Check sheet for the modelled part. Datum: model origin and axes. Units: mm. Round coordinates to 2 decimals unless told otherwise and drop trailing zeros. Order: outer loops, then holes, each group sorted by start corner. A loop starts at its lowest first (then second) coordinate and runs counter-clockwise, first axis right, second up.
Q1. Cross-section at B-B on x = -35. Record the cut outline in (y, z) (3 decimals), then the cut area to 3 significant figures.
Q2. Depth check by flat-ended pin: P1, Ø18.5, axis at x = 26.5, y = 14, coming from the +Z side. Enter the tip coordinate at first touch or a pass-through.
Q3. Scan lines: probe 1 along X at (y, z) = (-34.5, 3.75); probe 2 along X at (y, z) = (-36, 4.25); probe 3 along Y at (x, z) = (33, 4.75). Record each from-to range of solid material in increasing order.
Q4. Cross-section at A-A on y = 32.5. Record the cut outline in (x, z) (3 decimals).
Q5. Cross-section at C-C on z = 4.5. Give the number of separate pieces and of enclosed holes in the cut face, then the cut area to 3 significant figures.
from build123d import *

# Parameters (mm, degrees)
F1_DEPTH = 6.35
F3_DEPTH = 3.175


with BuildPart() as f1:
    # F0 (on Top) → F1 (new body)
    with BuildSketch(Plane.XY):
        with BuildLine():
            Line((44.45, 50.8), (-44.45, 50.8))
            ThreePointArc((-44.45, 50.8), (-48.940128, 48.940128), (-50.8, 44.45))
            Line((-50.8, 44.45), (-50.8, -44.45))
            ThreePointArc((-50.8, -44.45), (-48.940128, -48.940128), (-44.45, -50.8))
            Line((-44.45, -50.8), (44.45, -50.8))
            ThreePointArc((44.45, -50.8), (48.940128, -48.940128), (50.8, -44.45))
            Line((50.8, -44.45), (50.8, 44.45))
            ThreePointArc((50.8, 44.45), (48.940128, 48.940128), (44.45, 50.8))
        make_face()
    extrude(amount=F1_DEPTH)

    # F2 (on face) → F3 (cut)
    with BuildSketch(Plane.XY.offset(6.35)):
        with BuildLine():
            ThreePointArc((-24.847122, 30.86718), (-8.580237, 34.973614), (7.661782, 30.769903))
            ThreePointArc((7.661782, 30.769903), (-13.391629, 38.003846), (-33.371605, 28.186688))
            ThreePointArc((-33.371605, 28.186688), (-37.418416, 12.612971), (-27.426904, 0))
            ThreePointArc((-27.426904, 0), (-9.473393, 1.300027), (-4.446225, 18.584304))
            ThreePointArc((-4.446225, 18.584304), (-9.355194, 26.176966), (-18.170381, 28.186688))
            ThreePointArc((-18.170381, 28.186688), (-27.074817, 20.28871), (-24.843689, 8.597298))
            ThreePointArc((-24.843689, 8.597298), (-18.2062, 6.472593), (-12.664793, 10.699108))
            ThreePointArc((-12.664793, 10.699108), (-12.67809, 13.468506), (-14.519384, 15.537172))
            ThreePointArc((-14.519384, 15.537172), (-17.08667, 15.877181), (-18.994594, 14.12607))
            ThreePointArc((-18.994594, 14.12607), (-16.63705, 14.888107), (-14.519384, 13.601947))
            ThreePointArc((-14.519384, 13.601947), (-14.784471, 10.552305), (-17.140003, 8.597298))
            ThreePointArc((-17.140003, 8.597298), (-20.512291, 8.645462), (-23.187581, 10.699108))
            ThreePointArc((-23.187581, 10.699108), (-24.847122, 16.641338), (-22.353067, 22.284373))
            ThreePointArc((-22.353067, 22.284373), (-16.15161, 24.669828), (-10.003858, 22.149192))
            ThreePointArc((-10.003858, 22.149192), (-6.096197, 15.378887), (-7.423557, 7.675318))
            ThreePointArc((-7.423557, 7.675318), (-11.107583, 3.292778), (-16.414292, 1.143932))
            ThreePointArc((-16.414292, 1.143932), (-26.36106, 2.956962), (-32.86371, 10.699108))
            ThreePointArc((-32.86371, 10.699108), (-32.077882, 22.064039), (-24.847122, 30.86718))
        make_face()
        with BuildLine():
            ThreePointArc((-14.179834, -19.738191), (-10.270408, -12.968905), (-2.935242, -10.266648))
            ThreePointArc((-2.935242, -10.266648), (2.702162, -11.265838), (7.216472, -14.78716))
            ThreePointArc((7.216472, -14.78716), (10.619726, -24.307829), (7.166156, -33.810362))
            ThreePointArc((7.166156, -33.810362), (-3.069077, -38.81228), (-14.308201, -36.951829))
            ThreePointArc((-14.308201, -36.951829), (-25.997919, -24.91751), (-30.478409, -8.749654))
            ThreePointArc((-30.478409, -8.749654), (-26.216482, -30.599414), (-7.724586, -42.994002))
            ThreePointArc((-7.724586, -42.994002), (7.786055, -38.711784), (13.713452, -23.752396))
            ThreePointArc((13.713452, -23.752396), (3.61084, -8.854213), (-13.871366, -13.142696))
            ThreePointArc((-13.871366, -13.142696), (-17.992321, -21.190319), (-15.325198, -29.829356))
            ThreePointArc((-15.325198, -29.829356), (-4.033129, -33.591834), (4.976366, -25.813915))
            ThreePointArc((4.976366, -25.813915), (3.49767, -19.003328), (-2.933303, -16.317587))
            ThreePointArc((-2.933303, -16.317587), (-5.325023, -17.713801), (-6.195893, -20.342741))
            ThreePointArc((-6.195893, -20.342741), (-5.206707, -22.736081), (-2.736238, -23.512836))
            ThreePointArc((-2.736238, -23.512836), (-4.574954, -21.852161), (-4.519939, -19.375129))
            ThreePointArc((-4.519939, -19.375129), (-1.746329, -18.07988), (1.124523, -19.142327))
            ThreePointArc((1.124523, -19.142327), (2.768956, -22.086896), (2.328091, -25.430589))
            ThreePointArc((2.328091, -25.430589), (-1.98826, -29.838908), (-8.1223, -30.500511))
            ThreePointArc((-8.1223, -30.500511), (-13.288892, -26.322619), (-14.179834, -19.738191))
        make_face()
        with BuildLine():
            ThreePointArc((24.183692, -2.411001), (16.366605, -2.409982), (10.358799, 2.59133))
            ThreePointArc((10.358799, 2.59133), (8.405421, 7.97306), (9.19782, 13.643228))
            ThreePointArc((9.19782, 13.643228), (15.741335, 21.350867), (25.697555, 23.111254))
            ThreePointArc((25.697555, 23.111254), (35.146959, 16.748241), (39.155323, 6.084649))
            ThreePointArc((39.155323, 6.084649), (34.578156, -10.056104), (22.816627, -22.020249))
            ThreePointArc((22.816627, -22.020249), (39.60811, -7.404432), (41.096191, 14.807314))
            ThreePointArc((41.096191, 14.807314), (29.632361, 26.098813), (13.713452, 23.752396))
            ThreePointArc((13.713452, 23.752396), (5.862553, 7.554185), (18.317592, -5.441608))
            ThreePointArc((18.317592, -5.441608), (27.347515, -4.986647), (33.495579, 1.642667))
            ThreePointArc((33.495579, 1.642667), (31.107946, 13.303124), (19.867323, 17.216617))
            ThreePointArc((19.867323, 17.216617), (14.70853, 12.530736), (15.598096, 5.618478))
            ThreePointArc((15.598096, 5.618478), (18.003113, 4.245295), (20.715277, 4.80557))
            ThreePointArc((20.715277, 4.80557), (22.293377, 6.8589), (21.730832, 9.386766))
            ThreePointArc((21.730832, 9.386766), (21.212004, 6.964054), (19.039323, 5.773182))
            ThreePointArc((19.039323, 5.773182), (16.5308, 7.527575), (16.01548, 10.545029))
            ThreePointArc((16.01548, 10.545029), (17.743335, 13.441434), (20.85949, 14.73148))
            ThreePointArc((20.85949, 14.73148), (26.835382, 13.19757), (30.475367, 8.216137))
            ThreePointArc((30.475367, 8.216137), (29.440503, 1.652791), (24.183692, -2.411001))
        make_face()
    extrude(amount=-F3_DEPTH, mode=Mode.SUBTRACT)


solid = f1.part
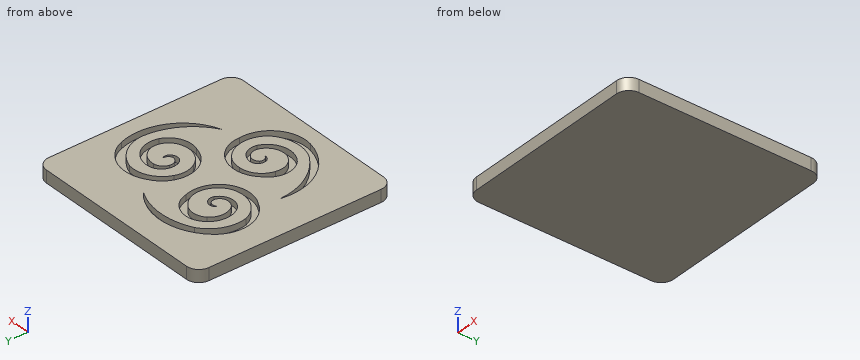
Results found:
1. outline: (-50.8, 0) - (50.8, 0) - (50.8, 6.35) - (26.003, 6.35) - (26.003, 3.175) - (6.671, 3.175) - (6.671, 6.35) - (-50.8, 6.35) - close
1. area: 584 mm2
2. P1: stops at z = 6.35
3. probe 1: x = -50.8 to -23.11, -17.8 to 6.41, 11.25 to 50.8
3. probe 2: x = -50.8 to -21.58, -15.78 to 4.4, 10.25 to 50.8
3. probe 3: y = -50.8 to -16.1, -12.52 to 0.51, 10.37 to 19.04, 24.6 to 50.8
4. outline: (-50.8, 0) - (50.8, 0) - (50.8, 6.35) - (5.51, 6.35) - (5.51, 3.175) - (4.025, 3.175) - (4.025, 6.35) - (-21.388, 6.35) - (-21.388, 3.175) - (-28.648, 3.175) - (-28.648, 6.35) - (-50.8, 6.35) - close
5. separate pieces: 1
5. enclosed holes: 3
5. area: 8,820 mm2
